Source: CAD feature listing. Evaluate the final solid. Frame: model axes, mm. A direction names the side the tool comes from. Give positions to 0.01 mm unless a question says otherwise; leave off trailing zeros. Loops run counter-clockwise (first coordinate to the right, second up) from the corner with the lowest first, then second, coordinate; pieces in that order, holes last.
```python
from build123d import *

# Parameters (mm, degrees)
F1_DEPTH          = 12.7
F2_R              = 6.35
F3_DEPTH          = 12.701
F8_R              = 7.62
F9_DEPTH          = 89.8035612107
F10_R             = 2.54
F11_DEPTH         = 6.35
F11_COPIES_COUNT  = 2
F11_COPIES_PITCH  = 14.929745
F11_COPIES1_COUNT = 2
F11_COPIES1_PITCH = 14.929745
F11_COPIES2_COUNT = 2
F11_COPIES2_PITCH = 24.156836
F11_COPIES3_COUNT = 2
F11_COPIES3_PITCH = 24.156836


# Not quite as in the source:
# - a pattern or mirror of a feature is missing from the dataset's text; its kind, count and spacing are read off the source's solid


with BuildPart() as f1:
    # F0 (on Top) → F1 (new body)
    with BuildSketch(Plane.XY):
        with BuildLine():
            Line((63.5, 0), (0, 0))
            Line((0, 0), (0, 12.7))
            ThreePointArc((0, 12.7), (-12.7, 25.4), (-25.4, 12.7))
            Line((-25.4, 12.7), (-25.4, -12.7))
            Line((-25.4, -12.7), (-12.7, -12.7))
            ThreePointArc((-12.7, -12.7), (-6.35, -19.05), (-12.7, -25.4))
            Line((-12.7, -25.4), (-25.4, -25.4))
            Line((-25.4, -25.4), (-25.4, -50.8))
            ThreePointArc((-25.4, -50.8), (-12.7, -63.5), (0, -50.8))
            Line((0, -50.8), (0, -38.1))
            Line((0, -38.1), (63.5, -38.1))
            Line((63.5, -38.1), (63.5, -50.8))
            ThreePointArc((63.5, -50.8), (76.2, -63.5), (88.9, -50.8))
            Line((88.9, -50.8), (88.9, 12.7))
            ThreePointArc((88.9, 12.7), (76.2, 25.4), (63.5, 12.7))
            Line((63.5, 12.7), (63.5, 0))
        make_face()
    extrude(amount=F1_DEPTH)

    # F2 (on face) → F3 (cut, through all)
    with BuildSketch(Plane.XY.offset(12.7)):
        with Locations((-12.7, 12.7)):
            Circle(F2_R)
        with Locations((76.2, 12.7)):
            Circle(F2_R)
        with Locations((76.2, -50.8)):
            Circle(F2_R)
        with Locations((-12.7, -50.8)):
            Circle(F2_R)
    extrude(amount=-F3_DEPTH, mode=Mode.SUBTRACT)

    # F6 (on face) → F7 (join, up to the next surface of F1)
    with BuildSketch(Plane(origin=(50.8, 0, 50.8), x_dir=(0, 1, 0), z_dir=(0.7071067812, 0, 0.7071067812))):
        with BuildLine():
            Line((-38.1, -18.9565367084), (-38.1, -53.8815367264))
            Line((-38.1, -53.8815367264), (0, -53.8815367264))
            Line((0, -53.8815367264), (0, -18.9565360082))
            ThreePointArc((0, -18.9565360082), (-19.0500003501, 0.0934632736), (-38.1, -18.9565367084))
        make_face()
    extrude(until=Until.NEXT, dir=(-0.7071067812, 0, -0.7071067812))

    # F8 (on face) → F9 (cut, through all)
    with BuildSketch(Plane(origin=(50.8, 0, 50.8), x_dir=(0, 1, 0), z_dir=(0.7071067812, 0, 0.7071067812))):
        with Locations((-19.05, -18.9565367264)):
            Circle(F8_R)
    extrude(amount=-F9_DEPTH, mode=Mode.SUBTRACT)

    # F10 (on face) → F11 (cut)
    with BuildSketch(Plane(origin=(50.8, 0, 50.8), x_dir=(0, 1, 0), z_dir=(0.7071067812, 0, 0.7071067812))):
        with Locations((-19.05, -6.2565367264)):
            Circle(F10_R)
    f11 = extrude(amount=-F11_DEPTH, mode=Mode.SUBTRACT)

    # F11_copies: F11 ×2
    with Locations(*[Vector(0.4156269378, -0.8090169944, -0.4156269378) * (i * F11_COPIES_PITCH) for i in range(1, F11_COPIES_COUNT)]):
        add(f11, mode=Mode.SUBTRACT)

    # F11_copies1: F11 ×2
    with Locations(*[Vector(0.4156269378, 0.8090169944, -0.4156269378) * (i * F11_COPIES1_PITCH) for i in range(1, F11_COPIES1_COUNT)]):
        add(f11, mode=Mode.SUBTRACT)

    # F11_copies2: F11 ×2
    with Locations(*[Vector(0.672498512, 0.3090169944, -0.672498512) * (i * F11_COPIES2_PITCH) for i in range(1, F11_COPIES2_COUNT)]):
        add(f11, mode=Mode.SUBTRACT)

    # F11_copies3: F11 ×2
    with Locations(*[Vector(0.672498512, -0.3090169944, -0.672498512) * (i * F11_COPIES3_PITCH) for i in range(1, F11_COPIES3_COUNT)]):
        add(f11, mode=Mode.SUBTRACT)


solid = f1.part
```
(1) Section A-A, the plane x = 76.2. Return the cut outline in (y, z), then the cut area to 3 significant figures.
A:
outline: (-63.5, 0) - (-57.15, 0) - (-57.15, 12.7) - (-63.5, 12.7) - close; (-44.45, 0) - (6.35, 0) - (6.35, 12.7) - (0, 12.7) - (0, 25.4) - (-38.1, 25.4) - (-38.1, 12.7) - (-44.45, 12.7) - close; (19.05, 0) - (25.4, 0) - (25.4, 12.7) - (19.05, 12.7) - close
area: 1,290 mm2
(2) Reachability of faces 1 (the flat face through (0, 6, 6)), 2 (the flat face through (0, -45, 6)), 3 (the flat face through (-19, -12.7, 6)) from +Z, -Z, +X, -X, +Y, -Y: full face, straight path, thin tool, end or side. Return the list, or none.
A:
face 1: +Z, -Z, +Y
face 2: +Z, -Z, -Y
face 3: +Z, -Z, -X
(3) Ray query, line 1 along Y through (x, z) = (76.2, 10); line 2 along X through (y, z) = (-50.5, 7); line 3 along Y through (x, z) = (80.5, 5). Return the intervals inside material, ascending.
A:
line 1: y = -63.5 to -57.15, -44.45 to 6.35, 19.05 to 25.4
line 2: x = -25.4 to -19.04, -6.36 to 0, 63.5 to 69.86, 82.54 to 88.9
line 3: y = -62.75 to -55.47, -46.13 to 8.03, 17.37 to 24.65
(4) Section C-C, the plane x = -10. Return the cut outline in (y, z), then the cut area to 3 significant figures.
A:
outline: (-63.21, 0) - (-56.55, 0) - (-56.55, 12.7) - (-63.21, 12.7) - close; (-45.05, 0) - (-24.8, 0) - (-24.8, 12.7) - (-45.05, 12.7) - close; (-13.3, 0) - (6.95, 0) - (6.95, 12.7) - (-13.3, 12.7) - close; (18.45, 0) - (25.11, 0) - (25.11, 12.7) - (18.45, 12.7) - close
area: 684 mm2
(5) Section D-D, the plane z = 8. Count the separate pieces of the cut face and the enclosed holes in it, then the cut area to 3 significant figures.
A:
separate pieces: 1
enclosed holes: 5
area: 5,670 mm2
(6) Section B-B, the plane y = 16.5. Return the cut outline in (x, z), then the cut area to 3 significant figures.
A:
outline: (-24.82, 0) - (-17.79, 0) - (-17.79, 12.7) - (-24.82, 12.7) - close; (-7.61, 0) - (-0.58, 0) - (-0.58, 12.7) - (-7.61, 12.7) - close; (64.08, 0) - (71.11, 0) - (71.11, 12.7) - (64.08, 12.7) - close; (81.29, 0) - (88.32, 0) - (88.32, 12.7) - (81.29, 12.7) - close
area: 357 mm2
(7) First-contact query: pin 1 (12.5 mm diameter, centred on x = 70, y = 11.5, fed in from +Z); pin 2 (1.5 mm diameter, centred on y = -10.5, z = 43.5, fed in from -X); pin 3 (18.5 mm diameter, centred on x = 40.5, z = 9.5, fed in from -Y). Flat tips, straight axial feed; report the tip coordinate or a pass-through.
A:
pin 1: stops at z = 12.7
pin 2: stops at x = 45.32
pin 3: stops at y = -38.1
(8) Mould query, pull axis Z, two halves, no side actions, for faces 4 (the flat face through (66.95, -26.55, 25.67)), 5 (the flat face through (63.5, -44, 6)), 6 (the cylindrical face through (31.921, -18.631, 32.047)). Classes: pulls with the +Z half, pulls with the -Z half, needs draft (parallel to the pull), parting line crosses it, or undercut.
A:
face 4: undercut
face 5: needs draft
face 6: pulls with the +Z half
